Read the model definition and answer for the solid it produces. Units are mm, in the model's axes. A direction names the side the tool comes from. Coordinates: 2 decimals unless noted, no trailing zeros. Order: outer loops, then holes, each group sorted by start corner. A loop starts at its lowest first (then second) coordinate and runs counter-clockwise, first axis right, second up. Notation, with made-up numbers: (55, 70.25) -> (69, 70.25) arc R25 ccw to (69, 99.25) -> close; hole circle Ø9 at (-24, 39). An arc over 180 degrees is marked (long way). Answer in a Markdown table with one row per item.
from build123d import *

# Parameters (mm, degrees)
F0_R     = 3.118101
F0_R_2   = 2.391899
F0_R_3   = 3.09485
F0_R_4   = 2.789347
F1_DEPTH = 2.54


with BuildPart() as f1:
    # F0 (on Front) → F1 (new body)
    with BuildSketch(Plane.XZ):
        with BuildLine():
            ThreePointArc((-42.396322, -48.584666), (-40.893992, -54.463207), (-34.939781, -55.630088))
            Line((-34.939781, -55.630088), (33.586267, -55.630088))
            ThreePointArc((33.586267, -55.630088), (36.404137, -54.636666), (37.975974, -52.095681))
            Line((37.975974, -52.095681), (37.975974, 37.562497))
            ThreePointArc((37.975974, 37.562497), (36.737459, 40.626378), (33.717722, 41.968942))
            Line((33.717722, 41.968942), (-41.97007, 63.180551))
            ThreePointArc((-41.97007, 63.180551), (-49.42771, 60.608198), (-49.647491, 52.722447))
            Line((-49.647491, 52.722447), (-20.833982, 17.965764))
            Line((-20.833982, 17.965764), (-42.396322, -48.584666))
        make_face()
        with Locations((-36.99355, -50.335164)):
            Circle(F0_R, mode=Mode.SUBTRACT)
        with Locations((33.586267, -51.136893)):
            Circle(F0_R_2, mode=Mode.SUBTRACT)
        Polygon((23.365004, -33.512361), (-30.987732, -33.512361), (-15.091307, 18.429529), align=None, mode=Mode.SUBTRACT)
        Polygon((28.063117, 34.616884), (32.164525, -32.620855), (-8.49389, 19.635132), align=None, mode=Mode.SUBTRACT)
        with Locations((-43.840472, 56.506539)):
            Circle(F0_R_3, mode=Mode.SUBTRACT)
        Polygon((22.234073, 40.242676), (-18.454095, 24.267845), (-39.46146, 50.549764), align=None, mode=Mode.SUBTRACT)
        with Locations((33.566951, 37.562497)):
            Circle(F0_R_4, mode=Mode.SUBTRACT)
    extrude(amount=F1_DEPTH)


solid = f1.part
Q1. Given pin 1 (6.5 mm diameter, centred on x = 33.57, z = 37.56, fed in from -Y); pin 2 (4 mm diameter, centred on x = 33.59, z = -51.14, fed in from +Y); pin 3 (1.3 mm diameter, centred on x = -13.5, y = -1.5, fed in from -Z), each flat-ended and moving along its own axis, determine where each tip first touches the part or whether it passes through.
Outcome:
| item | result |
|---|---|
| pin 1 | y = -2.54 |
| pin 2 | through |
| pin 3 | z = -55.63 |
Q2. For faces 4 (the face through (9.53, -1.25, 27.02)), 5 (the face through (13, 0, -9)), 6 (the face through (-35.442, -1.252, 35.587)), determine the directions among +Z, -Z, +X, -X, +Y, -Y from which every point of the face is accessible in a straight line to the end or side of a thin tool.
Outcome:
| item | result |
|---|---|
| face 4 | +Y, -Y |
| face 5 | +Z, -Z, +X, -X, +Y |
| face 6 | -X, +Y, -Y |
Q3. The part is cut by section C-C (x = -13.5). Write down the section's boundary in (y, z), then the cut area to 3 significant figures.
Outcome:
| item | result |
|---|---|
| outline | (-2.54, -55.63) -> (0, -55.63) -> (0, -33.51) -> (-2.54, -33.51) -> close; (-2.54, 16.28) -> (0, 16.28) -> (0, 26.21) -> (-2.54, 26.21) -> close; (-2.54, 46.21) -> (0, 46.21) -> (0, 55.2) -> (-2.54, 55.2) -> close |
| area | 104 mm² |
Q4. The part is cut by section B-B (x = 4). Write down the section's boundary in (y, z).
Outcome:
| item | result |
|---|---|
| outline | (-2.54, -55.63) -> (0, -55.63) -> (0, -33.51) -> (-2.54, -33.51) -> close; (-2.54, -7.36) -> (0, -7.36) -> (0, 3.58) -> (-2.54, 3.58) -> close; (-2.54, 24.76) -> (0, 24.76) -> (0, 33.08) -> (-2.54, 33.08) -> close; (-2.54, 43.29) -> (0, 43.29) -> (0, 50.3) -> (-2.54, 50.3) -> close |
Q5. The part is cut by section D-D (y = -1.9). Write down the section's boundary in (x, z) (1 decimal).
Outcome:
| item | result |
|---|---|
| outline | (-49.6, 52.7) -> (-20.8, 18) -> (-42.4, -48.6) arc R5.7 ccw to (-34.9, -55.6) -> (33.6, -55.6) arc R4.5 ccw to (38, -52.1) -> (38, 37.6) arc R4.4 ccw to (33.7, 42) -> (-42, 63.2) arc R6.9 ccw to start; hole circle Ø6.2 at (-43.8, 56.5); hole circle Ø6.2 at (-37, -50.3); hole (-39.5, 50.5) -> (-18.5, 24.3) -> (22.2, 40.2) -> close; hole (-31, -33.5) -> (23.4, -33.5) -> (-15.1, 18.4) -> close; hole (-8.5, 19.6) -> (32.2, -32.6) -> (28.1, 34.6) -> close; hole circle Ø5.6 at (33.6, 37.6); hole circle Ø4.8 at (33.6, -51.1) |
Q6. Consider line 1 (X direction, y = -1.95, z = -3); line 2 (X direction, y = -0.95, z = -49.5); line 3 (Z direction, x = 7.5, y = -1.8). Determine where each line is inside the solid, lowest interval first.
Outcome:
| item | result |
|---|---|
| line 1 | -27.63 to -21.65, 0.77 to 9.12, 30.36 to 37.98 |
| line 2 | -42.61 to -40, -33.99 to 31.84, 35.33 to 37.98 |
| line 3 | -55.63 to -33.51, -12.08 to -0.92, 26.19 to 34.46, 42.7 to 49.32 |
Q7. The part is cut by section A-A (z = 8.5). Write down the section's boundary in (x, y), then the cut area to 3 significant figures.
Outcome:
| item | result |
|---|---|
| outline | (-23.9, -2.54) -> (-18.13, -2.54) -> (-18.13, 0) -> (-23.9, 0) -> close; (-7.74, -2.54) -> (0.17, -2.54) -> (0.17, 0) -> (-7.74, 0) -> close; (29.66, -2.54) -> (37.98, -2.54) -> (37.98, 0) -> (29.66, 0) -> close |
| area | 55.9 mm² |
Q8. For a pull along X with two mould halves and no side action, classify faces 1 (the face through (-40.96, -1.25, -54.4)), 2 (the face through (2.175, -1.252, 32.367)), 3 (the face through (-1, -1, -55.63)) as pulls with the +X half, pulls with the -X half, needs draft (parallel to the pull), parting line crosses it, or undercut.
Outcome:
| item | result |
|---|---|
| face 1 | parting line crosses it |
| face 2 | undercut |
| face 3 | needs draft |
